Answer from the drawing. Dimensions are ordinates in mm from the lowest x, y and z of the part. A direction names the side the tool comes from. Round coordinates to 2 decimals unless told otherwise and drop trailing zeros. Write each loop counter-clockwise with the first axis right and the second up, starting at its lowest first coordinate (ties: lowest second). Pieces come first, ordered by that corner, then holes. Notation, with made-up numbers: (82, 35) - (93, 35) arc R16 cw to (93, 64) - close; hole circle Ø8 at (8.5, 55). An arc over 180 degrees is marked (long way). Answer in a Markdown table with one row per item.
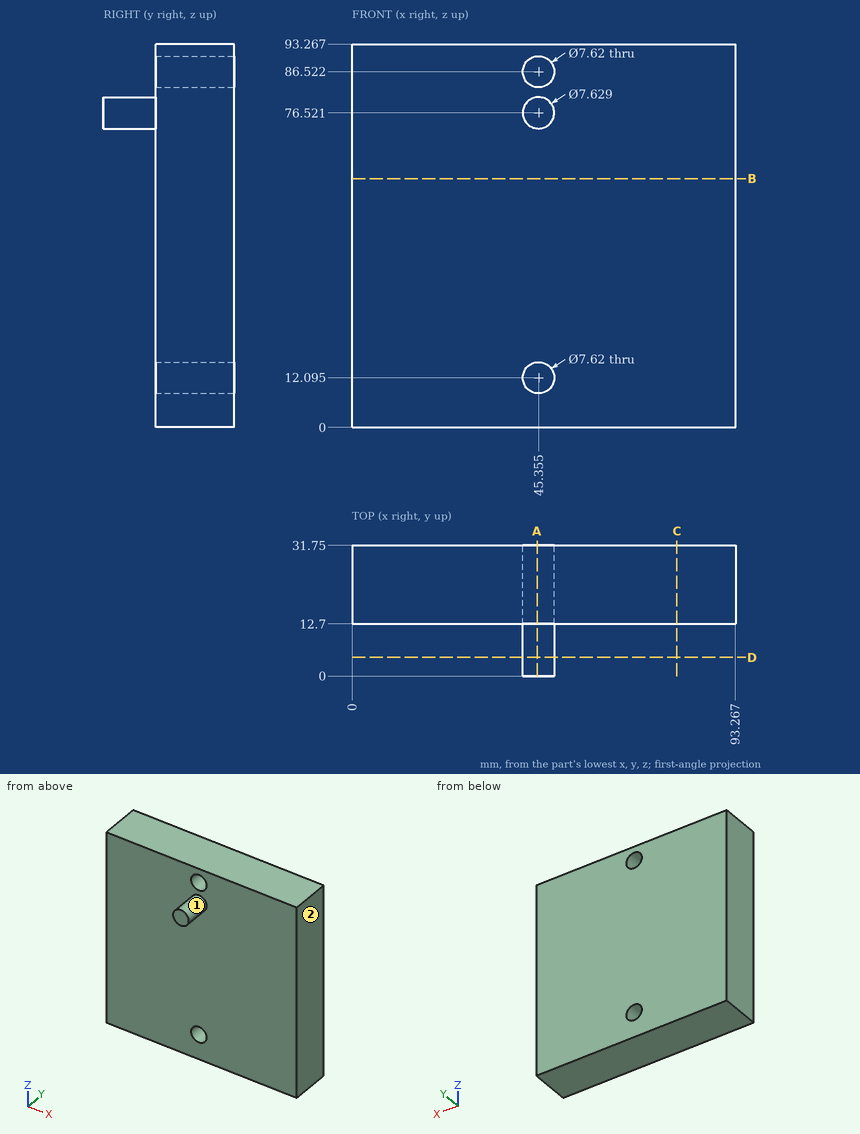
(1) Section A-A (x = 45) is taken. State how many separate pieces and enclosed holes the cut face has, and give its area (3 significant figures).
Checked values:
| item | result |
|---|---|
| separate pieces | 3 |
| enclosed holes | 0 |
| area | 1,580 mm2 |
(2) Section D-D (y = 4.5) is taken. Give the vertices of the cut face in (x, z) (1 decimal).
Checked values:
| item | result |
|---|---|
| outline | circle Ø7.6 at (45.4, 76.5) |
(3) For the marked faces 1 and 2, determine the directions among +Z, -Z, +X, -X, +Y, -Y from which every point of the face is accessible in a straight line to the end or side of a thin tool.
Checked values:
| item | result |
|---|---|
| face 1 | -Y |
| face 2 | +Z, -Z, +X, +Y, -Y |
(4) Section C-C (x = 79) is taken. Give the vertices of the cut face in (y, z), and give its area (3 significant figures).
Checked values:
| item | result |
|---|---|
| outline | (12.7, 0) - (31.75, 0) - (31.75, 93.27) - (12.7, 93.27) - close |
| area | 1,780 mm2 |
(5) Section B-B (z = 60.5) is taken. Give the vertices of the cut face in (x, y), and give its area (3 significant figures).
Checked values:
| item | result |
|---|---|
| outline | (0, 12.7) - (93.27, 12.7) - (93.27, 31.75) - (0, 31.75) - close |
| area | 1,780 mm2 |
(6) Flat-ended cylindrical pins translate along their axes: pin 1 (4 mm diameter, centred on y = 3, z = 79.5, fed in from +X); pin 2 (5 mm diameter, centred on x = 63.5, z = 52, fed in from -Y). Find the tip coordinate at first contact, or state that the pin passes through.
Checked values:
| item | result |
|---|---|
| pin 1 | stops at x = 49.04 |
| pin 2 | stops at y = 12.7 |
(7) Find the intervals of material crossed by line 1 (Z direction, x = 42.5, y = 19) (1 decimal); line 2 (Y direction, x = 39, z = 70); line 3 (X direction, y = 15, z = 12) (1 decimal), in increasing order.
Checked values:
| item | result |
|---|---|
| line 1 | z = 0 to 9.6, 14.6 to 84, 89 to 93.3 |
| line 2 | y = 12.7 to 31.75 |
| line 3 | x = 0 to 41.5, 49.2 to 93.3 |
